The model under review builds one solid part; all positions refer to its coordinate system, in mm. A direction names the side the tool comes from. Coordinates: 2 decimals unless noted, no trailing zeros. Write each loop counter-clockwise with the first axis right and the second up, starting at its lowest first coordinate (ties: lowest second). Pieces come first, ordered by that corner, then holes. Notation, with made-up numbers: M 9.25,-29.75 L 50.25,-29.75 A23 ccw 50.25,1.25 Z; hole C -30,-19.75 d3. An arc over 180 degrees is marked long. Answer as a JSON object with one key per item and string values.
```python
from build123d import *

# Parameters (mm, degrees)
F0_W     = 66.074446
F0_H     = 33.013113
F1_DEPTH = 12.7
F2_R     = 3.71087
F3_DEPTH = 6.35


with BuildPart() as f1:
    # F0 (on Top) → F1 (new body, symmetric)
    with BuildSketch(Plane.XY):
        with Locations((-33.037223, -41.1149)):
            Rectangle(F0_W, F0_H)
    extrude(amount=F1_DEPTH, both=True)

    # F2 (on face) → F3 (join)
    with BuildSketch(Plane.XY.offset(12.7)):
        with Locations((-8.831992, -41.570105)):
            Circle(F2_R)
    extrude(amount=F3_DEPTH)


solid = f1.part
```
(1) For faces 1 (the face through (-66.074, -41, 0)), 2 (the face through (-11.8, -43.8, 15.8)), list the 3-axis set-ups (+Z, -Z, +X, -X, +Y, -Y) from which the entire face can be reached by the end or side of a thin tool; tool diameter is ignored.
Results list:
{"face 1": "+Z, -Z, -X, +Y, -Y", "face 2": "+Z"}
(2) Add section C-C on z = 17. Give the boundary of the cut face in (x, y), and give its area (3 significant figures).
Results list:
{"outline": "C -8.83,-41.57 d7.42", "area": "43.3 mm²"}
(3) For pin 1 Ø10 at (x, y) = (-49.5, -46) entering from +Z, flat-tipped, find the tip position at first contact; note if it passes through.
Results list:
{"pin 1": "z = 12.7"}
(4) Add section D-D on y = -39.5. Give the boundary of the cut face in (x, z).
Results list:
{"outline": "M -66.07,-12.7 L 0,-12.7 L 0,12.7 L -5.75,12.7 L -5.75,19.05 L -11.91,19.05 L -11.91,12.7 L -66.07,12.7 Z"}
(5) Wall thickness on line 1 along Z through (x, y) = (-3.5, -49); line 2 along Y through (x, z) = (-12, 14): over which ranges is each line inside the solid? List them lowest first. Write a range as from..to.
Results list:
{"line 1": "-12.7..12.7", "line 2": "-43.5..-39.64"}
(6) Add section B-B on x = -55.5. Give the boundary of the cut face in (y, z), and give its area (3 significant figures).
Results list:
{"outline": "M -57.62,-12.7 L -24.61,-12.7 L -24.61,12.7 L -57.62,12.7 Z", "area": "839 mm²"}
(7) Add section A-A on y = -49. Give the boundary of the cut face in (x, z).
Results list:
{"outline": "M -66.07,-12.7 L 0,-12.7 L 0,12.7 L -66.07,12.7 Z"}
